Read the model definition and answer for the solid it produces. Units are mm, in the model's axes. A direction names the side the tool comes from. Give positions to 0.01 mm unless a question says otherwise; leave off trailing zeros. Order: outer loops, then holes, each group sorted by start corner. A loop starts at its lowest first (then second) coordinate and runs counter-clockwise, first axis right, second up. Notation, with made-up numbers: (-38, -32.75) - (-1, -32.75) arc R9 ccw to (-1, -17.75) - close; hole circle Ø10 at (-18, 1.25). An arc over 180 degrees is marked (long way). Use a Markdown table: item, result. Add a question column.
1. Consider L1, parallel to Y at x = -22, z = 7 (3 decimals); L2, parallel to X at y = 6.5, z = 5.5 (3 decimals); L3, parallel to X at y = 5, z = 3.75 (3 decimals). Determine where each line is inside the solid, lowest interval first.
2. For a pull along X with two mould halves and no side action, classify faces 1 (the flat face through (10.428, 0, 6)), 2 (the flat face through (-25, 10.795, 6)), 3 (the cylindrical face through (55.655, 9.115, 6.332)) as released by +X, released by -X, zero draft, split by the parting line, or undercut.
3. Flat-ended cylindrical pins translate along their axes: P1, Ø1.3, axis at x = -25.5, z = 7, coming from the +Y side (3 decimals); P2, Ø1.3, axis at y = 0.5, z = 6.5, coming from the +X side; P3, Ø6, axis at x = 16.5, y = 18, coming from the +Z side. Find the tip coordinate at first contact, or state that the pin passes through.
4. A cutting plane is placed at B-B on x = 14. Determine the outline of the cut face in (y, z) (3 decimals), and give its area (3 significant figures).
5. A cutting plane is placed at D-D on y = 13. Determine the outline of the cut face in (x, z), and give its area (3 significant figures).
6. A cutting plane is placed at C-C on x = -17. Determine the outline of the cut face in (y, z) (3 decimals), and give its area (3 significant figures).
7. Which of the six approach directions +Z, -Z, +X, -X, +Y, -Y give full straight-line access (tool end or side, diameter ignored) to faces 4 (the cylindrical face through (36.84, -9.42, 6.33)), 5 (the flat face through (-38, -10.795, 6)), 6 (the flat face through (-60.325, 0, 6)), 7 (the flat face through (-30.709, 9, 6)), 8 (the cylindrical face through (-19.052, 5.499, 6.332))?
8. A cutting plane is placed at A-A on z = 6.25. State how many separate pieces and enclosed holes the cut face has, and give its area (3 significant figures).
```python
from build123d import *

# Parameters (mm, degrees)
F0_R     = 3.81
F1_DEPTH = 5.08
F3_DEPTH = 2.54


with BuildPart() as f1:
    # F0 (on Top) → F1 (new body)
    with BuildSketch(Plane.XY):
        with BuildLine():
            Line((-60.325, -15.875), (53.975, -15.875))
            ThreePointArc((53.975, -15.875), (58.4651280605, -14.0151280605), (60.325, -9.525))
            Line((60.325, -9.525), (60.325, 9.525))
            ThreePointArc((60.325, 9.525), (58.4651280605, 14.0151280605), (53.975, 15.875))
            Line((53.975, 15.875), (-37.8134731769, 15.875))
            Line((-37.8134731769, 15.875), (-60.325, 15.875))
            Line((-60.325, 15.875), (-60.325, -15.875))
        make_face()
        with BuildLine():
            ThreePointArc((-37.8134731769, 15.875), (-74.4177446928, 17.9727124446), (-60.325, -15.875))
            Line((-60.325, -15.875), (-60.325, 15.875))
            Line((-60.325, 15.875), (-37.8134731769, 15.875))
        make_face()
        with Locations((-71.0623143972, 5.4617850045)):
            Circle(F0_R, mode=Mode.SUBTRACT)
    extrude(amount=F1_DEPTH)

    # F2 (on face) → F3 (join)
    with BuildSketch(Plane.XY.offset(5.08)):
        with BuildLine():
            Line((-55.2302619128, 10.795), (-60.325, 10.795))
            Line((-60.325, 10.795), (-60.325, -10.795))
            Line((-60.325, -10.795), (-55.245, -10.795))
            Line((-55.245, -10.795), (-55.245, 5.715))
            Line((-55.245, 5.715), (-50.165, 5.715))
            Line((-50.165, 5.715), (-50.165, -10.795))
            Line((-50.165, -10.795), (-45.085, -10.795))
            Line((-45.085, -10.795), (-45.085, 5.715))
            Line((-45.085, 5.715), (-41.275, 5.715))
            ThreePointArc((-41.275, 5.715), (-40.3769743879, 5.3430256121), (-40.005, 4.445))
            Line((-40.005, 4.445), (-40.005, -10.795))
            Line((-40.005, -10.795), (-34.925, -10.795))
            Line((-34.925, -10.795), (-34.925, -6.223))
            Line((-34.925, -6.223), (-34.925, -2.667))
            Line((-34.925, -2.667), (-34.925, 6.223))
            ThreePointArc((-34.925, 6.223), (-36.2641077964, 9.4558922036), (-39.497, 10.795))
            Line((-39.497, 10.795), (-55.2302619128, 10.795))
        make_face()
        with BuildLine():
            ThreePointArc((-30.353, 1.905), (-33.5858922036, 0.5658922036), (-34.925, -2.667))
            Line((-34.925, -2.667), (-34.925, -6.223))
            ThreePointArc((-34.925, -6.223), (-33.5858922036, -9.4558922036), (-30.353, -10.795))
            Line((-30.353, -10.795), (-13.208, -10.795))
            Line((-13.208, -10.795), (-13.208, -7.3516365111))
            Line((-13.208, -7.3516365111), (-13.208, 5.207))
            ThreePointArc((-13.208, 5.207), (-14.8446873067, 9.1583126933), (-18.796, 10.795))
            Line((-18.796, 10.795), (-30.7090226255, 10.795))
            Line((-30.7090226255, 10.795), (-30.7090226255, 6.223))
            Line((-30.7090226255, 6.223), (-20.828, 6.223))
            ThreePointArc((-20.828, 6.223), (-19.0319487758, 5.4790512242), (-18.288, 3.683))
            Line((-18.288, 3.683), (-18.288, 1.905))
            Line((-18.288, 1.905), (-30.353, 1.905))
        make_face()
        with BuildLine():
            ThreePointArc((-28.834547457, -5.6574139856), (-29.5493791419, -5.3578856134), (-29.845, -4.6414291305))
            Line((-29.845, -4.6414291305), (-29.845, -4.191))
            ThreePointArc((-29.845, -4.191), (-29.5474204897, -3.4725795103), (-28.829, -3.175))
            Line((-28.829, -3.175), (-18.288, -3.175))
            Line((-18.288, -3.175), (-18.288, -5.715))
            Line((-18.288, -5.715), (-28.834547457, -5.6574139856))
        make_face(mode=Mode.SUBTRACT)
        Polygon((-13.208, -7.3516365111), (-13.208, -10.795), (-9.4697934187, -10.795), (10.4281250387, 9.5132279851), (11.684, 10.795), (4.572, 10.795), align=None)
        with BuildLine():
            Line((11.684, 10.795), (10.4281250387, 9.5132279851))
            Line((10.4281250387, 9.5132279851), (10.4281250387, -10.795))
            Line((10.4281250387, -10.795), (11.684, -10.795))
            Line((11.684, -10.795), (28.078978887, -10.795))
            ThreePointArc((28.078978887, -10.795), (28.5957282879, -10.7686491822), (29.107116756, -10.6898701011))
            add(Edge.make_bspline(
                [(35.5372950435, -3.4511573613), (35.5250543244, -4.4661306449), (35.4891126843, -6.1377135055), (32.635648268, -10.1114027049), (29.9885608199, -10.5077053404), (29.107116756, -10.6898701011)],
                knots=[0.5939858484, 0.5939858484, 0.5939858484, 0.5939858484, 0.7105364175, 0.864635629, 0.978892706, 0.978892706, 0.978892706, 0.978892706], degree=3))
            Line((35.5372950435, -3.4511573613), (35.5372950435, -2.667))
            ThreePointArc((35.5372950435, -2.667), (35.5399098941, -2.512392897), (35.5477514548, -2.357962642))
            add(Edge.make_bspline(
                [(29.1883741966, 10.6813906829), (31.5964348364, 10.1488972227), (32.9847348448, 9.0372084423), (35.3473079701, 5.2056335604), (35.5537470863, 1.8236524058), (35.5559992426, -1.172556692), (35.5477514548, -2.357962642)],
                knots=[0.0105029487, 0.0105029487, 0.0105029487, 0.0105029487, 0.1576260779, 0.2979024518, 0.437582628, 0.5553822916, 0.5553822916, 0.5553822916, 0.5553822916], degree=3))
            ThreePointArc((29.1883741966, 10.6813906829), (28.518143702, 10.7832706341), (27.8403156543, 10.795))
            Line((27.8403156543, 10.795), (11.684, 10.795))
        make_face()
        with BuildLine():
            Line((27.1152709564, -5.715), (16.8622714295, -5.715))
            Line((16.8622714295, -5.715), (16.8622714295, 5.715))
            Line((16.8622714295, 5.715), (27.0222714295, 5.715))
            ThreePointArc((27.0222714295, 5.715), (28.3907110889, 5.3148534759), (29.3279882498, 4.2404904712))
            add(Edge.make_bspline(
                [(29.3279882498, 4.2404904712), (29.5322218703, 3.7985297904), (29.996949748, 2.7568174276), (30.1980545584, 1.7073743386), (30.6864836685, -0.4549893431), (29.9611913367, -2.9197379799), (29.5225347313, -4.0063798282), (29.4492436994, -4.177083447)],
                knots=[0.1184445178, 0.1184445178, 0.1184445178, 0.1184445178, 0.2235550269, 0.3756131932, 0.564595644, 0.8021758999, 0.8487485979, 0.8487485979, 0.8487485979, 0.8487485979], degree=3))
            ThreePointArc((29.4492436994, -4.177083447), (28.5128238256, -5.2959540253), (27.1152709564, -5.715))
        make_face(mode=Mode.SUBTRACT)
        with BuildLine():
            ThreePointArc((40.1092950435, 1.905), (36.9875755494, 0.6733669559), (35.5477514548, -2.357962642))
            add(Edge.make_bspline(
                [(35.5477514548, -2.357962642), (35.5450486122, -2.7464262804), (35.5413493806, -3.1149807203), (35.5372950435, -3.4511573613)],
                knots=[0.5553822916, 0.5553822916, 0.5553822916, 0.5553822916, 0.5939858484, 0.5939858484, 0.5939858484, 0.5939858484], degree=3))
            Line((35.5372950435, -3.4511573613), (35.5372950435, -6.223))
            ThreePointArc((35.5372950435, -6.223), (36.8764028399, -9.4558922036), (40.1092950435, -10.795))
            Line((40.1092950435, -10.795), (57.2480400174, -10.795))
            Line((57.2480400174, -10.795), (57.2480400174, 5.207))
            ThreePointArc((57.2480400174, 5.207), (55.6113527107, 9.1583126933), (51.6600400174, 10.795))
            Line((51.6600400174, 10.795), (46.4887204891, 10.795))
            Line((46.4887204891, 10.795), (41.9167204891, 10.795))
            Line((41.9167204891, 10.795), (41.9167204891, 6.223))
            Line((41.9167204891, 6.223), (41.9167204891, 5.715))
            Line((41.9167204891, 5.715), (49.6280400174, 5.715))
            ThreePointArc((49.6280400174, 5.715), (51.4240912417, 4.9710512242), (52.1680400174, 3.175))
            Line((52.1680400174, 3.175), (52.1680400174, 1.905))
            Line((52.1680400174, 1.905), (40.1092950435, 1.905))
        make_face()
        with BuildLine():
            ThreePointArc((40.622984476, -4.191), (40.9205639863, -3.4725795103), (41.638984476, -3.175))
            Line((41.638984476, -3.175), (52.1680400174, -3.175))
            Line((52.1680400174, -3.175), (52.1680400174, -5.715))
            Line((52.1680400174, -5.715), (41.6332798985, -5.715))
            ThreePointArc((41.6332798985, -5.715), (40.9168234157, -5.4193791419), (40.6172950435, -4.704547457))
            Line((40.6172950435, -4.704547457), (40.622984476, -4.191))
        make_face(mode=Mode.SUBTRACT)
        with BuildLine():
            add(Edge.make_bspline(
                [(35.5477514548, -2.357962642), (35.5450486122, -2.7464262804), (35.5413493806, -3.1149807203), (35.5372950435, -3.4511573613)],
                knots=[0.5553822916, 0.5553822916, 0.5553822916, 0.5553822916, 0.5939858484, 0.5939858484, 0.5939858484, 0.5939858484], degree=3))
            ThreePointArc((35.5477514548, -2.357962642), (35.5399098941, -2.512392897), (35.5372950435, -2.667))
            Line((35.5372950435, -2.667), (35.5372950435, -3.4511573613))
        make_face()
        Polygon((-2.9453631573, 5.715), (2.032, 10.795), (-11.176, 10.795), (-11.176, 5.715), align=None)
        Polygon((-1.9524302613, -5.715), (-6.9297934187, -10.795), (6.2782065813, -10.795), (6.2782065813, -5.715), align=None)
    extrude(amount=F3_DEPTH)


solid = f1.part
```
Output values:
| question | item | result |
|---|---|---|
| 1 | L1 | -10.795 to -5.695, -3.175 to 1.905, 6.223 to 10.795 |
| 1 | L2 | -60.325 to -34.933, -30.709 to -13.36, -11.176 to -2.176, 0.364 to 7.476, 10.428 to 34.449, 41.917 to 57.096 |
| 1 | L3 | -78.398 to -74.844, -67.28 to 60.325 |
| 2 | face 1 | undercut |
| 2 | face 2 | zero draft |
| 2 | face 3 | released by +X |
| 3 | P1 | y = 10.795 |
| 3 | P2 | x = 57.25 |
| 3 | P3 | z = 5.08 |
| 4 | outline | (-15.875, 0) - (15.875, 0) - (15.875, 5.08) - (10.795, 5.08) - (10.795, 7.62) - (-10.795, 7.62) - (-10.795, 5.08) - (-15.875, 5.08) - close |
| 4 | area | 216 mm² |
| 5 | outline | (-77.05, 0) - (59.29, 0) - (59.29, 5.08) - (-77.05, 5.08) - close |
| 5 | area | 693 mm² |
| 6 | outline | (-15.875, 0) - (15.875, 0) - (15.875, 5.08) - (10.499, 5.08) - (10.499, 7.62) - (-10.795, 7.62) - (-10.795, 5.08) - (-15.875, 5.08) - close |
| 6 | area | 215 mm² |
| 7 | face 4 | +Z, -Y |
| 7 | face 5 | +Z, +X, -X, -Y |
| 7 | face 6 | +Z, -X, +Y, -Y |
| 7 | face 7 | +Z, +Y |
| 7 | face 8 | +Z |
| 8 | separate pieces | 3 |
| 8 | enclosed holes | 3 |
| 8 | area | 1,670 mm² |
